Read the model definition and answer for the solid it produces. Units are mm, in the model's axes. A direction names the side the tool comes from. Coordinates: 2 decimals unless noted, no trailing zeros. Write each loop counter-clockwise with the first axis right and the second up, starting at its lowest first coordinate (ties: lowest second). Pieces come first, ordered by that corner, then holes.
Solid Edge part; units mm, degrees
sketch "Sketch1" plane through (0, 0, 0) normal (0, 0, 1) x (1, 0, 0)
  circle A0 centre (0, 0) radius 2.725
extrude "Protrusion1" add sketch "Sketch1" against normal blind 3
sketch "Sketch2" plane through (0, 0, 0) normal (0, 0, 1) x (1, 0, 0)
  line L0 (-0.7, -1.2124) -> (-1.05, -0.6062)
  line L1 (-1.4, 0) -> (-1.05, -0.6062)
  line L2 (-1.4, 0) -> (-1.05, 0.6062)
  line L3 (-0.7, 1.2124) -> (-1.05, 0.6062)
  line L4 (-0.7, 1.2124) -> (0, 1.2124)
  line L5 (0.7, 1.2124) -> (0, 1.2124)
  line L6 (0.7, 1.2124) -> (1.05, 0.6062)
  line L7 (1.4, 0) -> (1.05, 0.6062)
  line L8 (1.4, 0) -> (1.05, -0.6062)
  line L9 (0.7, -1.2124) -> (1.05, -0.6062)
  line L10 (0.7, -1.2124) -> (0, -1.2124)
  line L11 (-0.7, -1.2124) -> (0, -1.2124)
extrude "ExtrudedCutout_1" cut sketch "Sketch2" against normal blind 1.45
sketch "Sketch3" plane through (0, 0, -3) normal (0, 0, -1) x (1, 0, 0)
  circle A0 centre (0, 0) radius 1.45
extrude "ExtrudedProtrusion_2" add sketch "Sketch3" along normal blind 10
properties material "Stainless steel"
Item 1: For faces 4 (the flat face through (1, -1, 0)), 5 (the cylindrical face through (-1.45, 0.06, -7.93)), 6 (the flat face through (0, -1.212, -1)), determine the directions among +Z, -Z, +X, -X, +Y, -Y from which every point of the face is accessible in a straight line to the end or side of a thin tool.
Item 2: The part is cut by section C-C (z = -6.5). Give the vertices of the cut face in (x, y), and give its area (3 significant figures).
Item 3: Determine the mould class of faces 1 (the flat face through (0, 0, -1.45)), 2 (the cylindrical face through (2.6, 0.82, -1.48)), 3 (the flat face through (0, 0, -13)) for opening direction X: +X half, -X half, draft (parallel to the pull), parting line (faces both ways), or undercut.
Item 4: The part is cut by section D-D (x = -1.6). Give the vertices of the cut face in (y, z).
Item 5: Given pin 1 (2 mm diameter, centred on x = -2, z = -7, fed in from +Y); pin 2 (0.7 mm diameter, centred on x = 0, y = 0.5, fed in from +Z); pin 3 (1.5 mm diameter, centred on x = 1, z = -6.5, fed in from +Y), each flat-ended and moving along its own axis, determine where each tip first touches the part or whether it passes through.
Item 6: Find the intervals of material crossed by probe 1 along Z at (x, y) = (0, -1.85); probe 2 along Z at (x, y) = (0.3, -0.45); probe 3 along X at (y, z) = (-0.05, -1), in increasing order.
Item 7: The part is cut by section B-B (x = 0). Give the vertices of the cut face in (y, z) (3 decimals).
Item 8: The part is cut by section A-A (y = -0.8). Give the vertices of the cut face in (x, z), and give its area (3 significant figures).
Answer:
1. face 4: +Z, +X, -X, +Y, -Y
1. face 5: -Z
1. face 6: +Z
2. outline: circle Ø2.9 at (0, 0)
2. area: 6.61 mm2
3. face 1: undercut
3. face 2: parting line
3. face 3: draft
4. outline: (-2.21, -3) - (2.21, -3) - (2.21, 0) - (-2.21, 0) - close
5. pin 1: stops at y = 1.05
5. pin 2: stops at z = -1.45
5. pin 3: stops at y = 1.43
6. probe 1: z = -3 to 0
6. probe 2: z = -13 to -1.45
6. probe 3: x = -2.72 to -1.37, 1.37 to 2.72
7. outline: (-2.725, -3) - (-1.45, -3) - (-1.45, -13) - (1.45, -13) - (1.45, -3) - (2.725, -3) - (2.725, 0) - (1.212, 0) - (1.212, -1.45) - (-1.212, -1.45) - (-1.212, 0) - (-2.725, 0) - close
8. outline: (-2.6, -3) - (-1.21, -3) - (-1.21, -13) - (1.21, -13) - (1.21, -3) - (2.6, -3) - (2.6, 0) - (0.94, 0) - (0.94, -1.45) - (-0.94, -1.45) - (-0.94, 0) - (-2.6, 0) - close
8. area: 37.1 mm2
